Geometry: final body of the model. Coordinates: model frame, mm. Coordinates: 2 decimals unless noted, no trailing zeros. Order: outer loops, then holes, each group sorted by start corner. A loop starts at its lowest first (then second) coordinate and runs counter-clockwise, first axis right, second up. Notation, with made-up numbers: (39, 47) -> (97, 47) arc R16 ccw to (97, 70) -> close; hole circle Ø2 at (74, 80). An arc over 180 degrees is marked (long way). Answer in a Markdown table with one row per item. Add a question column.
1) Section query D-D on x = 34. Return the cut outline in (y, z).
2) Section query A-A on x = 0. Return the cut outline in (y, z).
3) Section query C-C on y = 0.6. Return the cut outline in (x, z), then the cut area to 3 significant figures.
4) Contact query for a flat-ended pin moving along its axis: P1, Ø4, axis at x = 44.17, z = 25.5, coming from the +Y side. Output: stop coordinate, or through.
5) Ray query, line 1 (Z direction, x = 0, y = 0.55); line 2 (X direction, y = 0.75, z = 25.5); line 3 (X direction, y = 0.6, z = 23.5). Return the intervals inside material, ascending. Write a range as from..to.
6) Section query B-B on z = -51. Return the cut outline in (x, y), then the cut area to 3 significant figures.
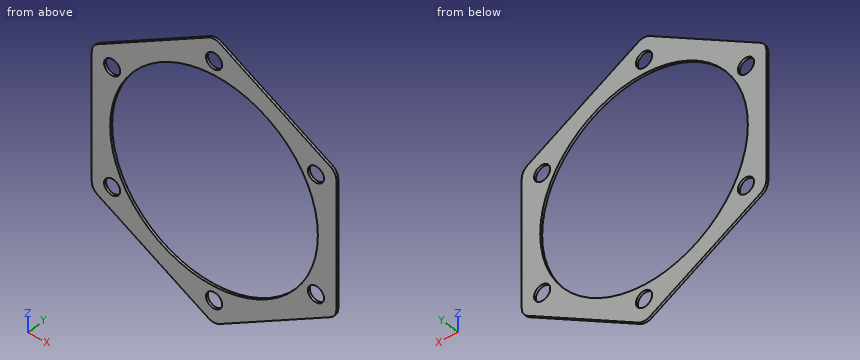
```python
from build123d import *

# Parameters (mm, degrees)
SKETCH1_R           = 45
SKETCH1_R_2         = 3.5
BOSS_EXTRUDE1_DEPTH = 1


with BuildPart() as part:
    # Sketch1 → Boss-Extrude1 (new body)
    with BuildSketch(Plane(origin=(0, 0, 0), x_dir=(1, 0, 0), z_dir=(0, 1, 0))):
        with BuildLine():
            Line((-2.5, 59.755752861), (-50.5, 32.04293994))
            ThreePointArc((-50.5, 32.04293994), (-52.330127019, 30.212812921), (-53, 27.712812921))
            Line((-53, 27.712812921), (-53, -27.712812921))
            ThreePointArc((-53, -27.712812921), (-52.330127019, -30.212812921), (-50.5, -32.04293994))
            Line((-50.5, -32.04293994), (-2.5, -59.755752861))
            ThreePointArc((-2.5, -59.755752861), (0, -60.425625842), (2.5, -59.755752861))
            Line((2.5, -59.755752861), (50.5, -32.04293994))
            ThreePointArc((50.5, -32.04293994), (52.330127019, -30.212812921), (53, -27.712812921))
            Line((53, -27.712812921), (53, 27.712812921))
            ThreePointArc((53, 27.712812921), (52.330127019, 30.212812921), (50.5, 32.04293994))
            Line((50.5, 32.04293994), (2.5, 59.755752861))
            ThreePointArc((2.5, 59.755752861), (0, 60.425625842), (-2.5, 59.755752861))
        make_face()
        Circle(SKETCH1_R, mode=Mode.SUBTRACT)
        with Locations((0, 51)):
            Circle(SKETCH1_R_2, mode=Mode.SUBTRACT)
        with Locations((44.167295593, 25.5)):
            Circle(SKETCH1_R_2, mode=Mode.SUBTRACT)
        with Locations((44.167295593, -25.5)):
            Circle(SKETCH1_R_2, mode=Mode.SUBTRACT)
        with Locations((0, -51)):
            Circle(SKETCH1_R_2, mode=Mode.SUBTRACT)
        with Locations((-44.167295593, -25.5)):
            Circle(SKETCH1_R_2, mode=Mode.SUBTRACT)
        with Locations((-44.167295593, 25.5)):
            Circle(SKETCH1_R_2, mode=Mode.SUBTRACT)
    extrude(amount=BOSS_EXTRUDE1_DEPTH)


solid = part.part
```
Result:
| question | item | result |
|---|---|---|
| 1 | outline | (0, -41.57) -> (1, -41.57) -> (1, -29.48) -> (0, -29.48) -> close; (0, 29.48) -> (1, 29.48) -> (1, 41.57) -> (0, 41.57) -> close |
| 2 | outline | (0, -60.43) -> (1, -60.43) -> (1, -54.5) -> (0, -54.5) -> close; (0, -47.5) -> (1, -47.5) -> (1, -45) -> (0, -45) -> close; (0, 45) -> (1, 45) -> (1, 47.5) -> (0, 47.5) -> close; (0, 54.5) -> (1, 54.5) -> (1, 60.43) -> (0, 60.43) -> close |
| 3 | outline | (-53, -27.71) arc R5 ccw to (-50.5, -32.04) -> (-2.5, -59.76) arc R5 ccw to (2.5, -59.76) -> (50.5, -32.04) arc R5 ccw to (53, -27.71) -> (53, 27.71) arc R5 ccw to (50.5, 32.04) -> (2.5, 59.76) arc R5 ccw to (-2.5, 59.76) -> (-50.5, 32.04) arc R5 ccw to (-53, 27.71) -> close; hole circle Ø7 at (-44.17, -25.5); hole circle Ø7 at (-44.17, 25.5); hole circle Ø90 at (0, 0); hole circle Ø7 at (0, -51); hole circle Ø7 at (0, 51); hole circle Ø7 at (44.17, -25.5); hole circle Ø7 at (44.17, 25.5) |
| 3 | area | 3,130 mm2 |
| 4 | P1 | through |
| 5 | line 1 | -60.43..-54.5, -47.5..-45, 45..47.5, 54.5..60.43 |
| 5 | line 2 | -53..-47.67, -40.67..-37.08, 37.08..40.67, 47.67..53 |
| 5 | line 3 | -53..-47.04, -41.3..-38.38, 38.38..41.3, 47.04..53 |
| 6 | outline | (-17.67, 0) -> (-3.5, 0) -> (-3.5, 1) -> (-17.67, 1) -> close; (3.5, 0) -> (17.67, 0) -> (17.67, 1) -> (3.5, 1) -> close |
| 6 | area | 28.3 mm2 |
